```python
from build123d import *

# Parameters (mm, degrees)
SKETCH_1_R               = 5
EXTRUDE_4_DEPTH          = 210
SKETCH_3_R               = 7.5
CUT_EXTRUDE_3_DEPTH      = 95
CUT_EXTRUDE_3_DEPTH_BACK = 95


with BuildPart() as part:
    # 草图1 → 凸台-拉伸4 (new body)
    with BuildSketch(Plane.XY):
        with BuildLine():
            ThreePointArc((0, 9), (0.292893219, 8.292893219), (1, 8))
            Line((1, 8), (85, 8))
            add(Edge.make_bspline(
                [(85, 8), (102.874129485, 7.751191804), (104.316426779, 7.753525507), (105.428932188, 5)],
                knots=[0, 0, 0, 0, 1, 1, 1, 1], degree=3))
            ThreePointArc((105.428932188, 5), (118.623724357, 3.169872981), (112.5, 15))
            Line((112.5, 15), (1, 15))
            ThreePointArc((1, 15), (0.292893219, 14.707106781), (0, 14))
            Line((0, 14), (0, 9))
        make_face()
        with Locations((112.5, 7.5)):
            Circle(SKETCH_1_R, mode=Mode.SUBTRACT)
    extrude(amount=EXTRUDE_4_DEPTH)

    # 草图3 → 切除-拉伸3 (cut, two sides)
    with BuildSketch(Plane(origin=(0, 0, 105), x_dir=(-1, 0, 0), z_dir=(0, 0, -1))) as cut_extrude_3_sk:
        with Locations((-112.5, 7.5)):
            Circle(SKETCH_3_R)
    extrude(amount=CUT_EXTRUDE_3_DEPTH, mode=Mode.SUBTRACT)
    extrude(cut_extrude_3_sk.sketch, amount=-CUT_EXTRUDE_3_DEPTH_BACK, mode=Mode.SUBTRACT)


solid = part.part
```
Verification items for the finished model (mm, model axes). A direction names the side the tool comes from. Give positions to 0.01 mm unless a question says otherwise; leave off trailing zeros. Order: outer loops, then holes, each group sorted by start corner. A loop starts at its lowest first (then second) coordinate and runs counter-clockwise, first axis right, second up. Notation, with made-up numbers: (77, -23) -> (115, -23) arc R12 ccw to (115, -8) -> close; hole circle Ø8 at (-40, -39.5). An arc over 180 degrees is marked (long way). One line per item, written item: value.
(1) Gauge pin test, flat end, axial feed: pin 1 (4 mm diameter, centred on y = 13.5, z = 156, fed in from +X). Record the tip position at first contact, or that the pin passes through.
Final values:
pin 1: x = 112.5
(2) Draft check along Z on faces 4 (the face through (118.5, 3, 204.9)), 5 (the face through (110.9, 2.6, 200)), 6 (the face through (59, 11, 210)). Enter one of: pulls with the +Z half, pulls with the -Z half, needs draft (parallel to the pull), parting line crosses it, or undercut.
Final values:
face 4: needs draft
face 5: undercut
face 6: pulls with the +Z half
(3) Sectioned sample at A-A on x = 49.5. Record the cut outline in (y, z).
Final values:
outline: (8, 0) -> (15, 0) -> (15, 210) -> (8, 210) -> close
(4) Scan lines: line 1 along Y through (x, z) = (73, 174.5); line 2 along Y through (x, z) = (112.5, 5.25); line 3 along X through (y, z) = (11, 84). Record each from-to range of solid material in increasing order. Write a range as [from, to].
Final values:
line 1: [8, 15]
line 2: [0, 2.5], [12.5, 15]
line 3: [0, 105.87]
(5) Tool access check on faces 1 (the face through (106.32, 11.75, 106.33)), 2 (the face through (59, 11, 0)), 3 (the face through (42, 8, 104)). Record the directions out of +Z, -Z, +X, -X, +Y, -Y that give a thin tool (end or side, any length) a straight path to the whole face; none if there is none.
Final values:
face 1: +X
face 2: -Z, +X, -X, +Y, -Y
face 3: +Z, -Z, -X, -Y
